Input: part model. Units: mm. Frame: model coordinates. Coordinates: 2 decimals unless noted, no trailing zeros. Loops run counter-clockwise (first coordinate to the right, second up) from the corner with the lowest first, then second, coordinate; pieces in that order, holes last.
(1) Contact query for flat-ended pins moving along their axis: P1, Ø1.4, axis at y = 94, z = 3, coming from the +X side; P2, Ø2, axis at x = -749.5, z = 2.5, coming from the +Y side; P3, Ø2.5, axis at x = -493, z = 2, coming from the +Y side. Output: stop coordinate, or through.
(2) Section A-A, the plane x = -89. Return loops of the section in (y, z), then the cut area to 3 significant figures.
(3) Mould query, pull axis Z, two halves, no side actions, for faces 1 (the face through (-432, 81, 4.826)), 2 (the face through (-766.512, 62.559, 2.379)), 3 (the face through (-432, 81, 0)). Classes: released by +Z, released by -Z, zero draft, split by the parting line, or undercut.
(4) Section B-B, the plane z = 1.65. Give the number of separate pieces and of enclosed holes in the cut face, then the cut area to 3 significant figures.
(5) Line query: L1, parallel to Y at x = -536.5, z = 2.75; L2, parallel to Y at x = -464, z = 2.9; L3, parallel to Y at x = -295, z = 1.5. Output: solid intervals per line, ascending.
(6) Section C-C, the plane y = 204.5. Return loops of the section in (x, z).
```python
from build123d import *

# Parameters (mm, degrees)
SKETCH1_R           = 3.3782
SKETCH1_R_2         = 8.000000002
SKETCH1_R_3         = 5.999999989
SKETCH1_R_4         = 5.999999988
SKETCH1_R_5         = 6.000000014
BOSS_EXTRUDE1_DEPTH = 4.826


with BuildPart() as part:
    # Sketch1 → Boss-Extrude1 (new body)
    with BuildSketch(Plane(origin=(0, 0, 0), x_dir=(-1, 0, 0), z_dir=(0, 0, -1))):
        with BuildLine():
            Line((534.606732, 122.174), (509.206732, 122.174))
            Line((509.206732, 122.174), (509.206732, 127))
            Line((509.206732, 127), (483.806732, 127))
            Line((483.806732, 127), (483.806732, 122.174))
            Line((483.806732, 122.174), (458.406732, 122.174))
            Line((458.406732, 122.174), (458.406732, 127))
            Line((458.406732, 127), (0, 127))
            Line((0, 127), (0, 101.6))
            Line((0, 101.6), (4.826, 101.6))
            Line((4.826, 101.6), (4.826, 76.2))
            Line((4.826, 76.2), (0, 76.2))
            Line((0, 76.2), (0, 50.8))
            Line((0, 50.8), (4.826, 50.8))
            Line((4.826, 50.8), (4.826, 25.4))
            Line((4.826, 25.4), (0, 25.4))
            Line((0, 25.4), (0, 0))
            Line((0, 0), (98.996246628, 0))
            ThreePointArc((98.996246628, 0), (104.569566166, -2.09646468), (109.562810755, -5.340623016))
            ThreePointArc((109.562810755, -5.340623016), (141.115933183, -16.717309509), (172.841249368, -5.830030532))
            ThreePointArc((172.841249368, -5.830030532), (180.737693875, -1.499037017), (189.618247276, 0))
            Line((189.618247276, 0), (308.116822983, 0))
            ThreePointArc((308.116822983, 0), (323.900159152, -3.422971591), (336.847489477, -13.076834684))
            ThreePointArc((336.847489477, -13.076834684), (357.417237927, -22.434421933), (377.979766443, -13.060980118))
            ThreePointArc((377.979766443, -13.060980118), (390.895425815, -3.419107464), (406.646288314, 0))
            Line((406.646288314, 0), (506.201416447, 0))
            ThreePointArc((506.201416447, 0), (507.045954934, -0.277722975), (507.560830812, -1.002483719))
            ThreePointArc((507.560830812, -1.002483719), (536.332746766, -22.486228157), (565.609234573, -1.69532427))
            ThreePointArc((565.609234573, -1.69532427), (567.234956908, 0.389735568), (569.808214418, 0.997019206))
            ThreePointArc((569.808214418, 0.997019206), (615.71405842, 2.124494779), (659.756153394, 15.121093757))
            Line((659.756153394, 15.121093757), (876.299999975, 111.343057166))
            Line((876.299999975, 111.343057166), (876.299999975, 136.743057212))
            Line((876.299999975, 136.743057212), (871.47400014, 136.743057212))
            Line((871.47400014, 136.743057212), (871.47400014, 162.143057105))
            Line((871.47400014, 162.143057105), (876.299999975, 162.143057105))
            Line((876.299999975, 162.143057105), (876.299999975, 187.543057156))
            Line((876.299999975, 187.543057156), (871.47400014, 187.543057156))
            Line((871.47400014, 187.543057156), (871.47400014, 212.943057198))
            Line((871.47400014, 212.943057198), (876.299999975, 212.943057198))
            Line((876.299999975, 212.943057198), (876.299999975, 238.343057355))
            Line((876.299999975, 238.343057355), (673.248258968, 143.658475478))
            ThreePointArc((673.248258968, 143.658475478), (636.589695375, 131.214569938), (598.106732, 127))
            Line((598.106732, 127), (534.606732, 127))
            Line((534.606732, 127), (534.606732, 122.174))
        make_face()
        with Locations((698.5, 63.500000033)):
            Circle(SKETCH1_R, mode=Mode.SUBTRACT)
        with Locations((704.85, 114.300000033)):
            Circle(SKETCH1_R, mode=Mode.SUBTRACT)
        with Locations((30.226, 25.400000033)):
            Circle(SKETCH1_R, mode=Mode.SUBTRACT)
        with Locations((622.3, 31.750000033)):
            Circle(SKETCH1_R, mode=Mode.SUBTRACT)
        with Locations((411.2514, 19.050000033)):
            Circle(SKETCH1_R, mode=Mode.SUBTRACT)
        with Locations((385.8514, 82.550000033)):
            Circle(SKETCH1_R, mode=Mode.SUBTRACT)
        with Locations((258.8514, 82.550000033)):
            Circle(SKETCH1_R, mode=Mode.SUBTRACT)
        with Locations((258.8514, 19.050000033)):
            Circle(SKETCH1_R, mode=Mode.SUBTRACT)
        with Locations((55.626, 88.900000033)):
            Circle(SKETCH1_R, mode=Mode.SUBTRACT)
        with Locations((609.6, 95.250000033)):
            Circle(SKETCH1_R, mode=Mode.SUBTRACT)
        with Locations((839.724, 162.143057153)):
            Circle(SKETCH1_R, mode=Mode.SUBTRACT)
        with Locations((141.506729012, 33.811031431)):
            Circle(SKETCH1_R_2, mode=Mode.SUBTRACT)
        with Locations((357.406729012, 4.829371893)):
            Circle(SKETCH1_R_3, mode=Mode.SUBTRACT)
        with Locations((536.696729012, 8.009371893)):
            Circle(SKETCH1_R_4, mode=Mode.SUBTRACT)
        with Locations((817.106729012, 132.869371893)):
            Circle(SKETCH1_R_5, mode=Mode.SUBTRACT)
    extrude(amount=-BOSS_EXTRUDE1_DEPTH)


solid = part.part
```
Report:
1. P1: stops at x = -4.83
1. P2: stops at y = 179.68
1. P3: stops at y = 127
2. outline: (0, 0) - (127, 0) - (127, 4.83) - (0, 4.83) - close
2. area: 613 mm2
3. face 1: released by +Z
3. face 2: zero draft
3. face 3: released by -Z
4. separate pieces: 1
4. enclosed holes: 15
4. area: 112,000 mm2
5. L1: y = -22.49 to 2.01, 14.01 to 127
5. L2: y = 0 to 122.17
5. L3: y = 0 to 127
6. outline: (-871.47, 0) - (-803.72, 0) - (-803.72, 4.83) - (-871.47, 4.83) - close
